Source: CAD feature listing. Evaluate the final solid. Frame: model axes, mm. A direction names the side the tool comes from. Give positions to 0.01 mm unless a question says otherwise; leave off trailing zeros. Write each loop counter-clockwise with the first axis right and the second up, starting at its lowest first coordinate (ties: lowest second). Pieces come first, ordered by that corner, then holes. Notation, with made-up numbers: (22.5, 38.5) - (32.5, 38.5) arc R29 cw to (32.5, 62.5) - close; hole circle Ø11 at (5, 54). An arc over 180 degrees is marked (long way). Answer as a JSON object with one key per item and string values. Group by question number.
from build123d import *

# Parameters (mm, degrees)
F0_R     = 17.5
F1_DEPTH = 15


with BuildPart() as f1:
    # F0 (on Top) → F1 (new body)
    with BuildSketch(Plane.XY):
        with BuildLine():
            Line((55.543554, 19.412428), (-99.456446, 19.412428))
            Line((-99.456446, 19.412428), (-99.456446, -5.587572))
            Line((-99.456446, -5.587572), (-99.456446, -35.587572))
            Line((-99.456446, -35.587572), (-89.456446, -35.587572))
            Line((-89.456446, -35.587572), (-89.456446, -5.587572))
            Line((-89.456446, -5.587572), (-79.456446, -5.587572))
            Line((-79.456446, -5.587572), (-79.456446, -20.587572))
            Line((-79.456446, -20.587572), (-71.456446, -20.587572))
            Line((-71.456446, -20.587572), (-71.456446, -5.587572))
            Line((-71.456446, -5.587572), (-61.456446, -5.587572))
            Line((-61.456446, -5.587572), (-54.882035, -22.152904))
            Line((-54.882035, -22.152904), (-48.307624, -5.587572))
            Line((-48.307624, -5.587572), (55.543554, -5.587572))
            ThreePointArc((55.543554, -5.587572), (123.235296, 6.912428), (55.543554, 19.412428))
        make_face()
        with Locations((88.235296, 6.912428)):
            Circle(F0_R, mode=Mode.SUBTRACT)
    extrude(amount=F1_DEPTH)


solid = f1.part
Q1. Draft query along X for faces 3 (the flat face through (-21, 19.412, 7)), 4 (the flat face through (-85, -5.588, 7)), 5 (the flat face through (-99.456, -8, 7)). Return one class per face: released by +X, released by -X, zero draft, split by the parting line, or undercut.
Q2. Section C-C on z = 9.5. Return the cut outline in (x, y), then the cut area to 3 significant figures.
Q3. First-contact query: pin 1 Ø1 at (x, z) = (92, 2.5) entering from +Y; pin 2 Ø4.5 at (x, z) = (14, 4.5) entering from -Y; pin 3 Ø7.5 at (x, z) = (-57, 7) entering from +Y. Flat tips, straight axial feed; report the tip coordinate or a pass-through.
Q4. Section D-D on y = -16.5. Return the cut outline in (x, z), then the cut area to 3 significant figures.
Q5. Section A-A on x = 83.5. Return the cut outline in (y, z), then the cut area to 3 significant figures.
Q6. Reachability of faces 1 (the flat face through (35, 4, 0)), 2 (the flat face through (-89.456, -21, 7)) from +Z, -Z, +X, -X, +Y, -Y: full face, straight path, thin tool, end or side. Return the list, or none.
Q7. Ray query, probe 1 along X at (y, z) = (6, 9.5); probe 2 along Y at (x, z) = (44, 4.5); probe 3 along X at (y, z) = (9, 11.5). Return the intervals inside material, ascending. Write a range as [from, to].
Q8. Section B-B on y = 12. Return the cut outline in (x, z), then the cut area to 3 significant figures.
Taken from the geometry:
{
 "1": {"face 3": "zero draft", "face 4": "undercut", "face 5": "released by -X"},
 "2": {"outline": "(-99.46, -35.59) - (-89.46, -35.59) - (-89.46, -5.59) - (-79.46, -5.59) - (-79.46, -20.59) - (-71.46, -20.59) - (-71.46, -5.59) - (-61.46, -5.59) - (-54.88, -22.15) - (-48.31, -5.59) - (55.54, -5.59) arc R35 ccw (long way) to (55.54, 19.41) - (-99.46, 19.41) - close; hole circle Ø35 at (88.24, 6.91)", "area": "7,250 mm²"},
 "3": {"pin 1": "stops at y = 41.76", "pin 2": "stops at y = -5.59", "pin 3": "stops at y = 19.41"},
 "4": {"outline": "(-99.46, 0) - (-89.46, 0) - (-89.46, 15) - (-99.46, 15) - close; (-79.46, 0) - (-71.46, 0) - (-71.46, 15) - (-79.46, 15) - close; (-57.13, 0) - (-52.64, 0) - (-52.64, 15) - (-57.13, 15) - close; (62.22, 0) - (114.25, 0) - (114.25, 15) - (62.22, 15) - close", "area": "1,120 mm²"},
 "5": {"outline": "(-27.77, 0) - (-9.93, 0) - (-9.93, 15) - (-27.77, 15) - close; (23.76, 0) - (41.59, 0) - (41.59, 15) - (23.76, 15) - close", "area": "535 mm²"},
 "6": {"face 1": "-Z, +X, -X, +Y, -Y", "face 2": "+Z, -Z, -Y"},
 "7": {"probe 1": "x = [-99.46, 70.76], [105.71, 123.22]", "probe 2": "y = [-5.59, 19.41]", "probe 3": "x = [-99.46, 70.86], [105.61, 123.17]"},
 "8": {"outline": "(-99.46, 0) - (71.49, 0) - (71.49, 15) - (-99.46, 15) - close; (104.98, 0) - (122.86, 0) - (122.86, 15) - (104.98, 15) - close", "area": "2,830 mm²"}
}
